Work out the finished part from the listing and answer in its coordinate system (mm). A direction names the side the tool comes from. Round coordinates to 2 decimals unless told otherwise and drop trailing zeros. Order: outer loops, then holes, each group sorted by start corner. A loop starts at its lowest first (then second) coordinate and runs counter-clockwise, first axis right, second up. Notation, with made-up numbers: (23.5, 75) -> (48.5, 75) arc R12 ccw to (48.5, 98) -> close; hole circle Ø1 at (-39.75, 41.25). An arc over 180 degrees is marked (long way). Use one line per item in the form item = value.
```python
from build123d import *

# Parameters (mm, degrees)
SKETCH_W               = 63
SKETCH_H               = 15.8
PAD_DEPTH              = 9.6
SKETCH001_W            = 60.6
SKETCH001_H            = 13.4
POCKET_DEPTH           = 8.6
SKETCH002_R            = 2.4
PAD001_DEPTH           = 1.8
LINEARPATTERN_COUNT    = 6
LINEARPATTERN_PITCH    = 11
SKETCH003_R            = 3.255
PAD002_DEPTH           = 8.6
LINEARPATTERN001_COUNT = 6
LINEARPATTERN001_PITCH = 9.4
SKETCH004_R            = 2.4
POCKET001_DEPTH        = 8.6
LINEARPATTERN002_COUNT = 6
LINEARPATTERN002_PITCH = 9.4


with BuildPart() as part:
    # Sketch → Pad (new body)
    with BuildSketch(Plane.XY):
        with Locations((5.290092, -4.615627)):
            Rectangle(SKETCH_W, SKETCH_H)
    extrude(amount=PAD_DEPTH)

    # Sketch001 → Pocket (cut)
    with BuildSketch(Plane(origin=(0, 0, 0), x_dir=(1, 0, 0), z_dir=(0, 0, -1))):
        with Locations((5.290092, 4.615627)):
            Rectangle(SKETCH001_W, SKETCH001_H)
    extrude(amount=-POCKET_DEPTH, mode=Mode.SUBTRACT)

    # Sketch002 → Pad001 (new body)
    with BuildSketch(Plane.XY.offset(9.6)):
        with Locations((-22.209908, -0.715627)):
            Circle(SKETCH002_R)
        with Locations((-22.209908, -8.515627)):
            Circle(SKETCH002_R)
    pad001 = extrude(amount=PAD001_DEPTH)

    # LinearPattern: Pad001 ×6
    with Locations(*[(i * LINEARPATTERN_PITCH, 0, 0) for i in range(1, LINEARPATTERN_COUNT)]):
        add(pad001)

    # Sketch003 → Pad002 (new body)
    with BuildSketch(Plane(origin=(0, 0, 8.6), x_dir=(1, 0, 0), z_dir=(0, 0, -1))):
        with Locations((-18.209908, 4.715627)):
            Circle(SKETCH003_R)
    pad002 = extrude(amount=PAD002_DEPTH)

    # LinearPattern001: Pad002 ×6
    with Locations(*[(i * LINEARPATTERN001_PITCH, 0, 0) for i in range(1, LINEARPATTERN001_COUNT)]):
        add(pad002)

    # Sketch004 → Pocket001 (cut)
    with BuildSketch(Plane(origin=(0, 0, 0), x_dir=(1, 0, 0), z_dir=(0, 0, -1))):
        with Locations((-18.209908, 4.715627)):
            Circle(SKETCH004_R)
    pocket001 = extrude(amount=-POCKET001_DEPTH, mode=Mode.SUBTRACT)

    # LinearPattern002: Pocket001 ×6
    with Locations(*[(i * LINEARPATTERN002_PITCH, 0, 0) for i in range(1, LINEARPATTERN002_COUNT)]):
        add(pocket001, mode=Mode.SUBTRACT)


solid = part.part
```
Item 1: A flat-ended cylindrical pin translates along its axis: P1, Ø4.5, axis at x = -18.21, y = -4.72, coming from the -Z side. Find the tip coordinate at first contact, or state that the pin passes through.
Findings:
P1 = 8.6
Item 2: Consider line 1 along X through (y, z) = (-11, 1); line 2 along Y through (x, z) = (-2, 7); line 3 along Y through (x, z) = (-12.5, 2.5). Determine where each line is inside the solid, lowest interval first.
Findings:
line_1 = -26.21 to -25.01, 35.59 to 36.79
line_2 = -12.52 to -11.32, -6.69 to -2.74, 2.08 to 3.28
line_3 = -12.52 to -11.32, 2.08 to 3.28
Item 3: The part is cut by section B-B, the plane x = 14. Give the vertices of the cut face in (y, z).
Findings:
outline = (-12.52, 0) -> (-11.32, 0) -> (-11.32, 8.6) -> (2.08, 8.6) -> (2.08, 0) -> (3.28, 0) -> (3.28, 9.6) -> (-12.52, 9.6) -> close
Item 4: The part is cut by section D-D, the plane x = 27.5. Give the vertices of the cut face in (y, z).
Findings:
outline = (-12.52, 0) -> (-11.32, 0) -> (-11.32, 8.6) -> (-7.7, 8.6) -> (-7.7, 0) -> (-6.74, 0) -> (-6.74, 8.6) -> (-2.69, 8.6) -> (-2.69, 0) -> (-1.73, 0) -> (-1.73, 8.6) -> (2.08, 8.6) -> (2.08, 0) -> (3.28, 0) -> (3.28, 9.6) -> (-12.52, 9.6) -> close
Item 5: Determine the mould class of faces 1 (the cylindrical face through (9.47, -2.373, 4.24)), 2 (the flat face through (-11, -8, 11.4)) for opening direction X: released by +X, released by -X, zero draft, split by the parting line, or undercut.
Findings:
face_1 = undercut
face_2 = zero draft
Item 6: The part is cut by section A-A, the plane z = 6. Give the number of separate pieces and of enclosed holes in the cut face, and give its area (3 significant figures).
Findings:
separate_pieces = 7
enclosed_holes = 7
area = 274 mm^2
Item 7: For faces 3 (the cylindrical face through (-9.92, -6.49, 10.49)), 4 (the flat face through (29, -5, 8.6)), 5 (the flat face through (0, -12, 0)), determine the directions among +Z, -Z, +X, -X, +Y, -Y from which every point of the face is accessible in a straight line to the end or side of a thin tool.
Findings:
face_3 = +Z
face_4 = -Z
face_5 = -Z, +X, -X, +Y, -Y
